Check sheet for the drawn part. Datum: minimum x, y, z corner. Units: mm. Give positions to 0.01 mm unless a question says otherwise; leave off trailing zeros. Write each loop counter-clockwise with the first axis right and the second up, starting at its lowest first coordinate (ties: lowest second). Pieces come first, ordered by that corner, then holes.
(1) Cross-section at D-D (x = 7.75). Record the boundary of the cut face in (y, z) (1 decimal).
(2) Depth check by flat-ended pin: P1, Ø1.5, axis at x = 8.5, z = 4, coming from the -Y side; P2, Ø1.5, axis at x = 4, y = 4.5, coming from the -Z side. Enter the tip coordinate at first touch or a pass-through.
(3) Cross-section at A-A (x = 4). Record the boundary of the cut face in (y, z).
(4) Thickness scan on line 1 along X through (y, z) = (4.5, 4) (1 decimal); line 2 along Z through (x, y) = (9.5, 3.5); line 3 along Y through (x, z) = (8, 4.5). Record the ranges inside material, lowest first.
(5) Cross-section at C-C (y = 1.25). Record the boundary of the cut face in (x, z).
(6) Mould release check, pull along X, two halves, no side actions. Record for the marked faces 1, 2 and 3: +X half, -X half, draft (parallel to the pull), parting line (faces both ways), or undercut.
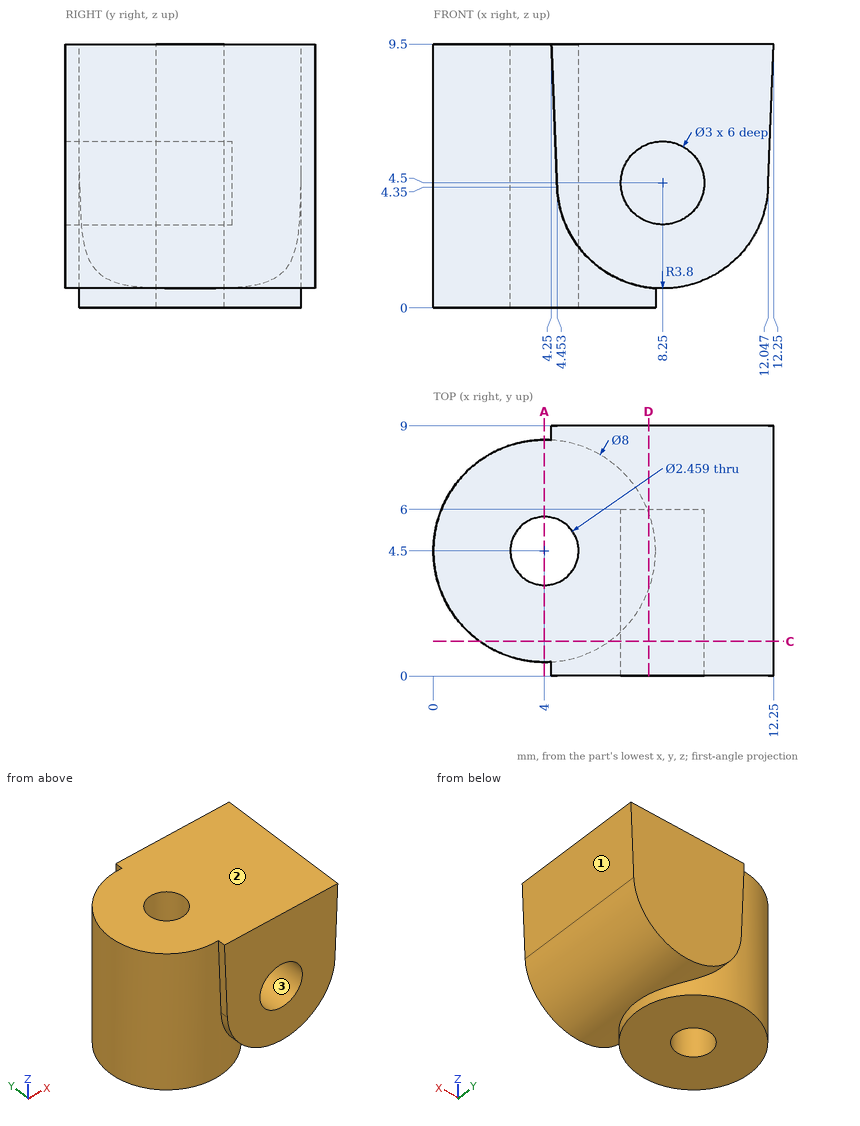
Reply:
1. outline: (0, 0.7) - (3.1, 0.7) - (3.1, 0) - (5.9, 0) - (5.9, 0.7) - (9, 0.7) - (9, 9.5) - (0, 9.5) - (0, 5.9) - (6, 5.9) - (6, 3.1) - (0, 3.1) - close
2. P1: stops at y = 6
2. P2: passes through
3. outline: (0.5, 0) - (3.27, 0) - (3.27, 9.5) - (0.5, 9.5) - close; (5.73, 0) - (8.5, 0) - (8.5, 9.5) - (5.73, 9.5) - close
4. line 1: x = 0 to 2.8, 5.2 to 6.8, 9.7 to 12
4. line 2: z = 0.91 to 3.67, 5.33 to 9.5
4. line 3: y = 6 to 9
5. outline: (1.67, 0) - (6.33, 0) - (6.33, 1.22) arc R3.8 ccw to (12.05, 4.35) - (12.25, 9.5) - (1.67, 9.5) - close; hole circle Ø3 at (8.25, 4.5)
6. face 1: +X half
6. face 2: draft
6. face 3: undercut
